```python
from build123d import *

# Parameters (mm, degrees)
SKETCH1_W                  = 25.4
SKETCH1_H                  = 25.4
SKETCH1_W_2                = 22.225
SKETCH1_H_2                = 22.225
BOSS_EXTRUDE1_DEPTH        = 812.8
F_7_0_201_DIAMETER_HOLE1_D = 5.1054
F_7_0_201_DIAMETER_HOLE2_D = 5.1054


with BuildPart() as part:
    # Sketch1 → Boss-Extrude1 (new body)
    with BuildSketch(Plane(origin=(0, 0, 0), x_dir=(1, 0, 0), z_dir=(0, 1, 0))):
        Rectangle(SKETCH1_W, SKETCH1_H)
        Rectangle(SKETCH1_W_2, SKETCH1_H_2, mode=Mode.SUBTRACT)
    extrude(amount=BOSS_EXTRUDE1_DEPTH)

    # #7 (0.201) Diameter Hole1 (through all)
    with Locations(Plane.XY.offset(12.7)):
        with Locations((0, 12.7), (0, 38.1), (0, 63.5), (0, 88.9), (0, 114.3), (0, 139.7), (0, 393.7), (0, 647.7), (0, 673.1), (0, 698.5), (0, 723.9), (0, 749.3), (0, 774.7), (0, 800.1)):
            Hole(F_7_0_201_DIAMETER_HOLE1_D / 2)

    # #7 (0.201) Diameter Hole2 (through all)
    with Locations(Plane(origin=(12.7, 0, 0), x_dir=(0, 0, -1), z_dir=(1, 0, 0))):
        with Locations((0, 38.1), (0, 190.5), (0, 342.9), (0, 469.9), (0, 622.3), (0, 774.7)):
            Hole(F_7_0_201_DIAMETER_HOLE2_D / 2)


solid = part.part
```
Can you work these out from the model? Positions are in its coordinate system, mm. A direction names the side the tool comes from. Coordinates: 2 decimals unless noted, no trailing zeros. Loops run counter-clockwise (first coordinate to the right, second up) from the corner with the lowest first, then second, coordinate; pieces in that order, holes last.
1) I need wall thicknesses on probe 1 along Z at (x, y) = (4.25, 722); probe 2 along Z at (x, y) = (12.15, 774.7). Which ranges of each line are inside material? Lowest first, please.
2) For pin 1 (10 mm diameter, centred on x = -1, z = 4, fed in from +Y), with a flat end and sliding along its axis, tell me the tip position at first contact or that it passes through.
3) Thinking about a two-plate mould opening in X: for faces 1 (the flat face through (-12.7, 401, 0)), 2 (the flat face through (0, 401, -11.112)), 3 (the flat face through (12.7, 401, 0)), 4 (the flat face through (0, 401, -12.7)), which applies, pulls with the +X half, pulls with the -X half, needs draft (parallel to the pull), parting line crosses it, or undercut?
4) Imagine slicing it at A-A on x = -7.25. List the corners of the cut face in (y, z) for me, plus the area to 3 significant figures.
5) Which directions (+Z, -Z, +X, -X, +Y, -Y) give clear straight access to the entire face, cutting with the end or side of a thin tool? Please do faces 5 (the flat face through (0, 401, 11.112)), 6 (the flat face through (-11.3, 0, -0.1)).
Completed:
1. probe 1: z = -12.7 to -11.11, 11.11 to 12.7
1. probe 2: z = -12.7 to -2.55, 2.55 to 12.7
2. pin 1: passes through
3. face 1: pulls with the -X half
3. face 2: undercut
3. face 3: pulls with the +X half
3. face 4: needs draft
4. outline: (0, -12.7) - (812.8, -12.7) - (812.8, -11.11) - (0, -11.11) - close; (0, 11.11) - (812.8, 11.11) - (812.8, 12.7) - (0, 12.7) - close
4. area: 2,580 mm2
5. face 5: +Y, -Y
5. face 6: +Z, -Z, +X, -X, -Y
